The listing builds one solid part. Answer for the finished solid, in the listing's coordinates (mm). Face numbers are marked on the shaded views. A direction names the side the tool comes from. Coordinates: 2 decimals unless noted, no trailing zeros. Order: outer loops, then holes, each group sorted by start corner. A loop starts at its lowest first (then second) coordinate and runs counter-clockwise, first axis right, second up. Notation, with made-up numbers: (1, 81) -> (35, 81) arc R24 ccw to (35, 92) -> close; hole circle Ø10 at (-35, 4). An arc over 180 degrees is marked (long way). Return JSON: item names as keys, results as strings.
from build123d import *

# Parameters (mm, degrees)
EXTRUDE_1_DEPTH = 3
SKETCH_2_R      = 3.2
EXTRUDE_2_DEPTH = 9
FILLET_1_R      = 0.2
EXTRUDE_3_DEPTH = 0.2
SKETCH_4_R      = 0.5
EXTRUDE_4_DEPTH = 0.4
SKETCH_5_W      = 1
SKETCH_5_H      = 0.25
EXTRUDE_5_DEPTH = 2


with BuildPart() as part:
    # 草图1 → 凸台-拉伸1 (new body)
    with BuildSketch(Plane.XY):
        with BuildLine():
            Line((1, 0), (11, 0))
            ThreePointArc((11, 0), (11.707106781, -0.292893219), (12, -1))
            Line((12, -1), (12, -11))
            ThreePointArc((12, -11), (11.707106781, -11.707106781), (11, -12))
            Line((11, -12), (1, -12))
            ThreePointArc((1, -12), (0.292893219, -11.707106781), (0, -11))
            Line((0, -11), (0, -1))
            ThreePointArc((0, -1), (0.292893219, -0.292893219), (1, 0))
        make_face()
    extrude(amount=EXTRUDE_1_DEPTH)

    # 草图2 → 凸台-拉伸2 (add)
    with BuildSketch(Plane.XY.offset(3)):
        with Locations(Location((6, -6, 0), (0, 0, 180))):
            Circle(SKETCH_2_R)
    extrude(amount=EXTRUDE_2_DEPTH)

    # 圆角1
    fillet_1_edges = [part.edges().sort_by_distance(p)[0] for p in [
        (9.2, -6, 12),
    ]]
    fillet(fillet_1_edges, radius=FILLET_1_R)

    # 草图3 → 凸台-拉伸3 (add)
    with BuildSketch(Plane.XY.offset(3)):
        with BuildLine():
            Line((1.5, -0.5), (10.5, -0.5))
            ThreePointArc((10.5, -0.5), (11.207106781, -0.792893219), (11.5, -1.5))
            Line((11.5, -1.5), (11.5, -10.5))
            ThreePointArc((11.5, -10.5), (11.207106781, -11.207106781), (10.5, -11.5))
            Line((10.5, -11.5), (1.5, -11.5))
            ThreePointArc((1.5, -11.5), (0.792893219, -11.207106781), (0.5, -10.5))
            Line((0.5, -10.5), (0.5, -1.5))
            ThreePointArc((0.5, -1.5), (0.792893219, -0.792893219), (1.5, -0.5))
        make_face()
    extrude(amount=EXTRUDE_3_DEPTH)

    # 草图4 → 凸台-拉伸4 (add)
    with BuildSketch(Plane.XY.offset(3.2)):
        with Locations((2, -2)):
            Circle(SKETCH_4_R)
        with Locations(Location((10, -2, 0), (0, 0, 180))):
            Circle(SKETCH_4_R)
        with Locations((10, -10)):
            Circle(SKETCH_4_R)
        with Locations(Location((2, -10, 0), (0, 0, 180))):
            Circle(SKETCH_4_R)
    extrude(amount=EXTRUDE_4_DEPTH)

    # 草图5 → 凸台-拉伸5 (add)
    with BuildSketch(Plane(origin=(0, 0, 0), x_dir=(-1, 0, 0), z_dir=(0, 0, -1))):
        with Locations((-3.5, -11.875)):
            Rectangle(SKETCH_5_W, SKETCH_5_H)
        with Locations((-8.5, -11.875)):
            Rectangle(SKETCH_5_W, SKETCH_5_H)
        with Locations((-8.5, -0.125)):
            Rectangle(SKETCH_5_W, SKETCH_5_H)
        with Locations((-3.5, -0.125)):
            Rectangle(SKETCH_5_W, SKETCH_5_H)
    extrude(amount=EXTRUDE_5_DEPTH)


solid = part.part
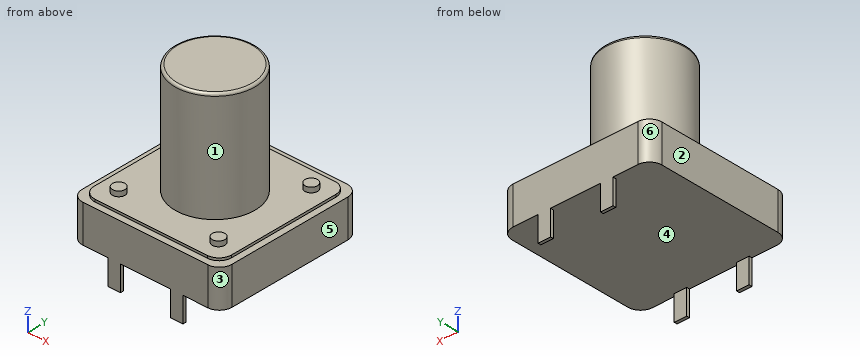
1. Consider line 1 (Y direction, x = 8.75, z = -1); line 2 (Z direction, x = 3, y = -5.5); line 3 (Z direction, x = 11, y = -5.5). Determine where each line is inside the solid, lowest interval first. Write a range as from..to.
Answer block:
{"line 1": "y = -12..-11.75, -0.25..0", "line 2": "z = 0..12", "line 3": "z = 0..3.2"}
2. Determine the mould class of the marked faces 3, 4, 5 and 6 for opening direction Y: pulls with the +Y half, pulls with the -Y half, needs draft (parallel to the pull), parting line crosses it, or undercut.
Answer block:
{"face 3": "pulls with the -Y half", "face 4": "undercut", "face 5": "needs draft", "face 6": "pulls with the +Y half"}
3. Each of these flat-tipped pins is pushed along its axis until it touches: pin 1 Ø2 at (y, z) = (-6.5, 7.5) entering from -X; pin 2 Ø1.1 at (x, y) = (2, -2) entering from +Z; pin 3 Ø1 at (x, z) = (6, 5.5) entering from -Y; pin 4 Ø4 at (x, y) = (2.5, -9) entering from +Z. Where does it stop, or does it pass through?
Answer block:
{"pin 1": "stops at x = 2.8", "pin 2": "stops at z = 3.6", "pin 3": "stops at y = -9.2", "pin 4": "stops at z = 12"}
4. The part is cut by section C-C on y = -6. Give the vertices of the cut face in (x, z).
Answer block:
{"outline": "(0, 0) -> (12, 0) -> (12, 3) -> (11.5, 3) -> (11.5, 3.2) -> (9.2, 3.2) -> (9.2, 11.8) arc R0.2 ccw to (9, 12) -> (3, 12) arc R0.2 ccw to (2.8, 11.8) -> (2.8, 3.2) -> (0.5, 3.2) -> (0.5, 3) -> (0, 3) -> close"}
5. The part is cut by section D-D on z = 5.25. Give the vertices of the cut face in (x, y), and give its area (3 significant figures).
Answer block:
{"outline": "circle Ø6.4 at (6, -6)", "area": "32.2 mm2"}
6. For the marked faces 1 and 2, determine the directions among +Z, -Z, +X, -X, +Y, -Y from which every point of the face is accessible in a straight line to the end or side of a thin tool.
Answer block:
{"face 1": "+Z", "face 2": "+Z, -Z, -X, +Y, -Y"}
7. The part is cut by section A-A on z = -1. Give the vertices of the cut face in (x, y).
Answer block:
{"outline": "(3, -12) -> (4, -12) -> (4, -11.75) -> (3, -11.75) -> close; (3, -0.25) -> (4, -0.25) -> (4, 0) -> (3, 0) -> close; (8, -12) -> (9, -12) -> (9, -11.75) -> (8, -11.75) -> close; (8, -0.25) -> (9, -0.25) -> (9, 0) -> (8, 0) -> close"}
8. The part is cut by section B-B on x = 10. Give the vertices of the cut face in (y, z), and give its area (3 significant figures).
Answer block:
{"outline": "(-12, 0) -> (0, 0) -> (0, 3) -> (-0.5, 3) -> (-0.5, 3.2) -> (-1.5, 3.2) -> (-1.5, 3.6) -> (-2.5, 3.6) -> (-2.5, 3.2) -> (-9.5, 3.2) -> (-9.5, 3.6) -> (-10.5, 3.6) -> (-10.5, 3.2) -> (-11.5, 3.2) -> (-11.5, 3) -> (-12, 3) -> close", "area": "39.0 mm2"}
